Can you work these out from the model? Positions are in its coordinate system, mm. A direction names the side the tool comes from. Coordinates: 2 decimals unless noted, no trailing zeros. Order: outer loops, then holes, each group sorted by start corner. A loop starts at its lowest first (then second) coordinate and runs counter-clockwise, first axis right, second up.
Autodesk Inventor part; units mm, degrees
ref_plane "YZ Plane" through (0, 0, 0) normal (1, 0, 0) x (0, 1, 0)
ref_plane "XZ Plane" through (0, 0, 0) normal (0, 1, 0) x (-1, 0, 0)
ref_plane "XY Plane" through (0, 0, 0) normal (0, 0, 1) x (1, 0, 0)
sketch "Boceto15" plane through (0, 0, 0) normal (1, 0, 0) x (0, 1, 0)
  line L0 (24.65, 10) -> (-24.65, 10)
  line L1 (-24.65, 10) -> (-24.65, -10)
  line L2 (-24.65, -10) -> (24.65, -10)
  line L3 (24.65, -10) -> (24.65, 10)
  line L4 (0, -2.1261) -> (0, 0)
  line L5 (0, 0) -> (1.5481, 0)
  dimension "d52" = 49.3
  dimension "d53" = 20
extrude "Extrusión12" add sketch "Boceto15" along normal blind 5
sketch "Boceto16" plane through (5, 0, 0) normal (1, 0, 0) x (0, 0, -1)
  circle A0 centre (3.5, -14.65) radius 1.5
  line L0 (10, -24.65) -> (10, 24.65)
  line L1 (-10, -24.65) -> (10, -24.65)
  circle A1 centre (3.5, 7.35) radius 1.5
  point P0 (0, 0)
  dimension "d56" = 6.5
  dimension "d57" = 10
  dimension "d58" = 3
  dimension "d59" = 3
  dimension "d60" = 32
  dimension "d61" = 6.5
extrude "Extrusión13" cut sketch "Boceto16" against normal through all
sketch "Boceto17" plane through (0, -24.65, -10) normal (0, -1, 0) x (1, 0, 0)
  line L0 (5, 20) -> (5, 0)
  line L1 (5, 20) -> (16, 20)
  line L2 (16, 20) -> (16, 15)
  line L3 (16, 15) -> (5, 15)
  line L4 (5, 15) -> (5, 20)
  line L5 (16, 15) -> (21, 15)
  line L6 (21, 15) -> (21, 31)
  line L7 (21, 31) -> (16, 31)
  line L8 (16, 31) -> (16, 15)
  line L9 (21, 31) -> (41, 31)
  line L10 (41, 31) -> (41, 26)
  line L11 (41, 26) -> (21, 26)
  line L12 (21, 26) -> (21, 31)
  point P0 (0, 10)
  dimension "d64" = 11
  dimension "d65" = 5
  dimension "d66" = 5
  dimension "d67" = 16
  dimension "d91" = 20
  dimension "d92" = 5
extrude "Extrusión14" add sketch "Boceto17" against normal up to surface (49.3 mm away)
sketch "Boceto18" plane through (0, -24.65, 10) normal (0, 0, 1) x (1, 0, 0)
  circle A0 centre (10, 24.3) radius 2
  line L0 (0, 0) -> (16, 0)
  line L1 (0, 49.3) -> (0, 0)
  point P0 (0, 24.65)
  dimension "d70" = 24.3
  dimension "d71" = 10
  dimension "d127" = 4
extrude "Extrusión15" cut sketch "Boceto18" against normal up to surface (5 mm away)
sketch "Boceto19" plane through (5, 0, 0) normal (1, 0, 0) x (0, 0, -1)
  line L0 (10, -24.65) -> (10, 24.65)
  line L1 (10, -22) -> (7, -22)
  line L2 (7, -22) -> (7, -16)
  line L3 (7, -16) -> (10, -16)
  line L4 (10, -16) -> (10, -22)
  line L5 (10, 9) -> (7, 9)
  line L6 (7, 9) -> (7, 15)
  line L7 (7, 15) -> (10, 15)
  line L8 (10, 15) -> (10, 9)
  line L9 (7, 12) -> (8.4797, 12)
  line L10 (7, -19) -> (9.1788, -19)
  line L11 (-5, -24.65) -> (10, -24.65)
  point P0 (0, 0)
  dimension "d74" = 5.65
  dimension "d75" = 6
  dimension "d76" = 6
  dimension "d77" = 31
  dimension "d78" = 3
extrude "Extrusión16" cut sketch "Boceto19" against normal through all
sketch "Boceto20" plane through (21, -24.65, 5) normal (0, 0, -1) x (-1, 0, 0)
  line L0 (16, 49.3) -> (16, 0)
  line L1 (5, 0) -> (5, 49.3)
  line L2 (2, 0) -> (2, 49.3)
  line L3 (16, 8.65) -> (16, 33.65)
  line L4 (2, 28.65) -> (16, 28.65)
  line L5 (16, 28.65) -> (16, 13.65)
  line L6 (16, 13.65) -> (0, 13.65)
  line L7 (2, 13.65) -> (2, 28.65)
  line L8 (21, 33.65) -> (16, 33.65)
  point P0 (2, 13.65)
  dimension "d85" = 5
  dimension "d86" = 15
  dimension "d94" = 14
extrude "Extrusión17" add sketch "Boceto20" along normal up to surface (15 mm away)
sketch "Boceto21" plane through (0, -16, -10) normal (0, 0, -1) x (-1, 0, 0)
  circle A0 centre (-10, 15.65) radius 2
  circle A1 centre (-14, 15.65) radius 2
  line L0 (-14, 15.65) -> (-14.5246, 15.65)
  line L1 (-10, 15.65) -> (-9.1195, 15.65)
  line L2 (-21, -8.65) -> (-21, 40.65)
  point P0 (0, 16)
  dimension "d87" = 4
  dimension "d106" = 7
extrude "Extrusión18" cut sketch "Boceto21" against normal blind 7 contours A1
sketch "Boceto22" plane through (0, -24.65, -10) normal (0, -1, 0) x (1, 0, 0)
  line L0 (21, 15) -> (21, 26)
  line L1 (21, 13.5) -> (41, 13.5)
  line L2 (41, 13.5) -> (41, 8.5)
  line L3 (41, 8.5) -> (21, 8.5)
  line L4 (21, 8.5) -> (21, 13.5)
  line L5 (21, 26) -> (41, 26)
  line L6 (16, 31) -> (16, 20)
  line L7 (21, 8.5) -> (16, 8.5)
  line L8 (16, 8.5) -> (16, 20)
  line L9 (16, 20) -> (21, 20)
  line L10 (21, 20) -> (21, 8.5)
  point P0 (0, 10)
  dimension "d95" = 5
  dimension "d96" = 12.5
extrude "Extrusión19" add sketch "Boceto22" against normal up to surface (49.3 mm away)
sketch "Boceto24" plane through (41, -24.65, 3.5) normal (1, 0, 0) x (0, 0, -1)
  line L0 (-17.5, 0) -> (-17.5, 49.3)
  line L1 (5, 0) -> (5, 49.3)
  line L2 (-17.5, 0) -> (5, 0)
  line L3 (5, 0) -> (5, 49.3)
  line L4 (5, 49.3) -> (-17.5, 49.3)
  line L5 (-17.5, 49.3) -> (-17.5, 0)
  point P0 (3.5, 24.65)
extrude "Extrusión21" add sketch "Boceto24" along normal blind 5
sketch "Boceto26" plane through (46, -24.65, 3.5) normal (1, 0, 0) x (0, 0, -1)
  line L0 (-17.5, 49.3) -> (-6.5, 49.3)
  line L1 (5, 28.65) -> (5, 49.3)
  line L2 (-17.5, 49.3) -> (5, 49.3)
  line L3 (5, 49.3) -> (5, 43.3)
  line L4 (5, 43.3) -> (-17.5, 43.3)
  line L5 (-17.5, 43.3) -> (-17.5, 49.3)
  point P0 (3.5, 24.65)
  point P1 (-6.5, 49.3)
  dimension "d111" = 6
extrude "Extrusión23" cut sketch "Boceto26" against normal up to surface (30 mm away)
sketch "Boceto25" plane through (19, -11, -10) normal (1, 0, 0) x (0, 0, -1)
  line L0 (-15, -13.65) -> (0, -13.65)
  line L1 (-8.5, -13.65) -> (-8.5, 0)
  line L2 (0, -13.65) -> (-8.5, -13.65)
  line L3 (-8.5, -13.65) -> (-8.5, -6.65)
  line L4 (-8.5, -6.65) -> (0, -6.65)
  line L5 (0, -6.65) -> (0, -13.65)
  line L6 (-8.5, 0) -> (0, 0)
  line L7 (0, 0) -> (-3, 0)
  line L8 (-3, 0) -> (-3, -6.65)
  line L9 (-3, -6.65) -> (0, -6.65)
  line L10 (0, -6.65) -> (0, 0)
  line L11 (-8.5, 15) -> (-8.5, 29.65)
  line L12 (-8.5, 29.65) -> (0, 29.65)
  line L13 (0, 29.65) -> (0, 22.65)
  line L14 (0, 22.65) -> (-8.5, 22.65)
  line L15 (-8.5, 22.65) -> (-8.5, 29.65)
  line L16 (-8.5, 15) -> (0, 15)
  line L17 (0, 22.65) -> (-3, 22.65)
  line L18 (-3, 22.65) -> (-3, 15)
  line L19 (-3, 15) -> (0, 15)
  line L20 (0, 15) -> (0, 22.65)
  point P0 (-10, 11)
  point P1 (0, -6.65)
  point P2 (-3, 0)
  dimension "d107" = 7
  dimension "d108" = 3
  dimension "d114" = 7
extrude "Extrusión22" add sketch "Boceto25" against normal up to surface (14 mm away) contours L1 L4 L5 L0 | L4 L8 L6 L10 | L11 L12 L13 L14 | L18 L14 L20 L16
sketch "Boceto27" plane through (0, -24.65, -10) normal (0, -1, 0) x (1, 0, 0)
  line L0 (19, 0) -> (19, 8.5)
  line L1 (46, 8.5) -> (46, 31)
  line L2 (19, 0) -> (46, 0)
  line L3 (46, 0) -> (46, 8.5)
  line L4 (46, 8.5) -> (19, 8.5)
  line L5 (19, 8.5) -> (19, 0)
  point P0 (0, 10)
extrude "Extrusión24" add sketch "Boceto27" against normal up to surface (43.3 mm away)
sketch "Boceto23" plane through (16, -24.65, 21) normal (0, 0, 1) x (1, 0, 0)
  circle A0 centre (15.15, 21.15) radius 2.5
  line L0 (0, 0) -> (0, 49.3)
  line L1 (25, 0) -> (0, 0)
  point P0 (-16, 24.65)
  dimension "d99" = 15.15
  dimension "d100" = 21.15
  dimension "d103" = 5
extrude "Extrusión20" cut sketch "Boceto23" against normal through all
sketch "Boceto28" plane through (5, 24.65, -10) normal (0, 0, -1) x (-1, 0, 0)
  circle A0 centre (-26.15, -28.15) radius 2.5
  circle A1 centre (-26.15, -28.15) radius 3.5
  point P0 (5, -24.65)
  dimension "d117" = 7
extrude "Extrusión25" cut sketch "Boceto28" against normal blind 7
sketch "Boceto29" plane through (46, -24.65, 3.5) normal (1, 0, 0) x (0, 0, -1)
  circle A0 centre (7, 10) radius 1.5
  circle A1 centre (7, 32) radius 1.5
  circle A2 centre (7, 32) radius 3.5
  circle A3 centre (7, 10) radius 3.5
  point P0 (3.5, 24.65)
  dimension "d120" = 7
  dimension "d121" = 7
extrude "Extrusión26" cut sketch "Boceto29" against normal up to surface (30 mm away) contours A0 | A1 | A2 | A3
chamfer "Chaflán1" distance 1 angle 45 1 edges at (28.65, -3.5, 3.5)
equation "\"d59\" = d58"
equation "\"d61\" = d56"
equation "\"d76\" = d75"
properties part number "Base Idler Izq" material "Resina fenólica"
1. Imagine slicing it at A-A on x = 31.15. Please give me the cut outline in (y, z), then the cut area to 3 significant figures.
Completed:
outline: (-24.65, -10) - (-7, -10) - (-7, -3) - (-6, -3) - (-6, 2.5) - (-7, 3.5) - (-24.65, 3.5) - close; (-24.65, 16) - (-6, 16) - (-6, 21) - (-24.65, 21) - close; (-1, -3) - (0, -3) - (0, -10) - (18.65, -10) - (18.65, 3.5) - (0, 3.5) - (-1, 2.5) - close; (-1, 16) - (18.65, 16) - (18.65, 21) - (-1, 21) - close; hole circle Ø7 at (-14.65, -3.5); hole circle Ø7 at (7.35, -3.5)
area: 617 mm2
2. I'm going to push flat-ended pins straight in: pin 1 (8 mm diameter, centred on x = 12, z = -3.5, fed in from +Y); pin 2 (4 mm diameter, centred on y = 22.5, z = 7.5, fed in from +X); pin 3 (1 mm diameter, centred on y = -17, z = 12.5, fed in from -X). Where does each tip first touch, or does it pass through?
Completed:
pin 1: stops at y = 18.65
pin 2: stops at x = 16
pin 3: stops at x = 16
3. Imagine slicing it at B-B on z = 8.5. Please give me the cut outline in (x, y).
Completed:
outline: (0, -24.65) - (21, -24.65) - (21, 18.65) - (16, 18.65) - (16, 24.65) - (0, 24.65) - close; (41, -24.65) - (46, -24.65) - (46, 18.65) - (41, 18.65) - close; hole circle Ø4 at (10, -0.35)
4. Please list where these lines run through material, in increasing order: probe 1 along Z at (x, y) = (32, 14); probe 2 along X at (y, z) = (-20, 15); probe 3 along Z at (x, y) = (9, -17.5).
Completed:
probe 1: z = -10 to 3.5, 16 to 21
probe 2: x = 16 to 21, 41 to 46
probe 3: z = -10 to -7, 5 to 10
5. On a 3-axis mill with a long thin cutter (end or side, diameter ignored), from which of +Z, -Z, +X, -X, +Y, -Y can I reach the whole of each face in a straight line? I mean faces 1 (the flat face through (16, -18, 2)), 2 (the flat face through (17, 11, -1.5)), 3 (the flat face through (3, 15, -8)), 4 (the flat face through (14, 0, -3)). Say none if no direction works.
Completed:
face 1: -Y
face 2: none
face 3: -Z, -X
face 4: -Z
6. Imagine slicing it at C-C on y = -3.5. Please give me the cut outline in (x, z), then the cut area to 4 significant figures.
Completed:
outline: (0, -10) - (27.65, -10) - (27.65, -3) - (28.65, -3) - (28.65, 2.5) - (27.65, 3.5) - (21, 3.5) - (21, 16) - (28.65, 16) - (28.65, 21) - (16, 21) - (16, 10) - (0, 10) - close; (33.65, -3) - (34.65, -3) - (34.65, -10) - (46, -10) - (46, 21) - (33.65, 21) - (33.65, 16) - (41, 16) - (41, 3.5) - (34.65, 3.5) - (33.65, 2.5) - close
area: 892.5 mm2
7. Imagine slicing it at D-D on x = 39. Please give me the cut outline in (y, z).
Completed:
outline: (-24.65, -10) - (18.65, -10) - (18.65, 3.5) - (-24.65, 3.5) - close; (-24.65, 16) - (18.65, 16) - (18.65, 21) - (-24.65, 21) - close; hole circle Ø7 at (-14.65, -3.5); hole circle Ø7 at (7.35, -3.5)
8. Thinking about a two-plate mould opening in Z: for faces 5 (the flat face through (3, -16, -8)), 6 (the flat face through (10, 0, 5)), 7 (the flat face through (41, -3, 10)), which applies, pulls with the +Z half, pulls with the -Z half, needs draft (parallel to the pull), parting line crosses it, or undercut?
Completed:
face 5: needs draft
face 6: pulls with the +Z half
face 7: undercut
